Design review of the part built by this model. Coordinates are the model's own, in mm. A direction names the side the tool comes from. Give positions to 0.01 mm unless a question says otherwise; leave off trailing zeros. Loops run counter-clockwise (first coordinate to the right, second up) from the corner with the lowest first, then second, coordinate; pieces in that order, holes last. Notation, with made-up numbers: (26, 59.5) - (76, 59.5) arc R7 cw to (76, 70.5) - close; hole circle Ø1 at (-14.75, -26.75). An arc over 180 degrees is marked (long way). Put each result on its own line as item: value. Start each with the question number.
```python
from build123d import *

# Parameters (mm, degrees)
F1_DEPTH = 50
F2_R     = 5.08
F3_T     = -1


# Not quite as in the source:
# - a shell that OpenCascade refuses in one call is made with other operations: the cavity is built on its own and cut out


with BuildPart() as f1:
    # F0 (on Right) → F1 (new body)
    with BuildSketch(Plane.YZ):
        Polygon((40.6505316496, -75.3882825375), (40.6505316496, 73.1709599495), (-17.738416791, 15.5211091042), (-18.8470706344, -75.3882825375), align=None)
    extrude(amount=F1_DEPTH)

    # F2
    f2_edges = [f1.edges().sort_by_distance(p)[0] for p in [
        (50, -18.292744, -29.933587),
        (50, 11.456057, 44.346035),
        (25, -17.738417, 15.521109),
        (0, 11.456057, 44.346035),
        (25, -18.847071, -75.388283),
        (0, -18.292744, -29.933587),
    ]]
    fillet(f2_edges, radius=F2_R)

    # F3: a shell. OpenCascade refuses it in one call, so the cavity is built on its own and cut out:
    # the body offset inwards by the wall thickness, plus a prism from it out through each open face.
    f3_core = offset(f1.part, amount=F3_T, mode=Mode.PRIVATE)
    f3_exits = [f3_core.faces().sort_by_distance(p)[0] for p in [
        (49, 15.243523, -16.834061),
    ]]
    add(f3_core, mode=Mode.SUBTRACT)
    extrude(f3_exits, amount=-F3_T, mode=Mode.SUBTRACT)


solid = f1.part
```
Item 1: For P1, Ø4, axis at y = 3, z = -30, coming from the +X side; P2, Ø14.5, axis at x = 22, y = 10, coming from the +Z side; P3, Ø5, axis at x = 41.5, y = 19.5, coming from the +Z side, all flat-tipped, find the tip position at first contact; note any pin that passes through.
Item 2: For L1, parallel to X at y = 1, z = 15.5; L2, parallel to Y at x = 3, z = -62.5; L3, parallel to Y at x = 45, z = 9.5, list the stretches that pass through material, from the lowest coordinate up. Write a range as from..to.
Item 3: Mouldability with a two-part tool opening along Z and no side actions: class faces 1 (the cylindrical face through (1.53, 12.82, 43.66)), 2 (the flat face through (25, 13, -75.388)), 3 (the flat face through (25, 39.651, -3)) as pulls with the +Z half, pulls with the -Z half, needs draft (parallel to the pull), parting line crosses it, or undercut.
Item 4: Consider section A-A (x = 27). State the section outline as (y, z) points.
Item 5: Machinability: for faces 4 (the cylindrical face through (1.528, -16.864, -31.585)), 5 (the cylindrical face through (25.28, -16.43, 14.99)), 6 (the cylindrical face through (25.279, -17.348, 15.385)), 7 (the flat face through (1, 13, -19)), which of the approach directions +Z, -Z, +X, -X, +Y, -Y give a long, thin tool a straight path to every point of the face, cutting with its end or side? Answer none if there is none.
Geometry says:
1. P1: stops at x = 1
1. P2: stops at z = 50.07
1. P3: stops at z = 54.76
2. L1: x = 0..1
2. L2: y = -18.24..-17.12, 39.65..40.65
2. L3: y = -17.81..-16.81, 39.65..40.65
3. face 1: pulls with the +Z half
3. face 2: pulls with the -Z half
3. face 3: undercut
4. outline: (-18.78, -70.25) arc R5.08 ccw to (-13.7, -75.39) - (40.65, -75.39) - (40.65, 73.17) - (-16.25, 16.99) arc R5.08 ccw to (-17.76, 13.43) - close; hole (-17.78, -70.26) arc R4.08 ccw to (-13.7, -74.39) - (39.65, -74.39) - (39.65, 70.78) - (-15.55, 16.28) arc R4.08 ccw to (-16.76, 13.42) - close
5. face 4: +Z, -X, -Y
5. face 5: none
5. face 6: +Z, +X, -X, -Y
5. face 7: +X
